Autodesk Inventor part; units mm, degrees
ref_plane "YZ Plane" through (0, 0, 0) normal (1, 0, 0) x (0, 1, 0)
ref_plane "XZ Plane" through (0, 0, 0) normal (0, 1, 0) x (-1, 0, 0)
ref_plane "XY Plane" through (0, 0, 0) normal (0, 0, 1) x (1, 0, 0)
sketch "Sketch1" plane through (0, 0, 0) normal (1, 0, 0) x (0, 1, 0)
  line L0 (0, 0) -> (3.175, 0)
  line L1 (3.175, 0) -> (3.175, -21.59)
  line L2 (3.175, -21.59) -> (0, -21.59)
  line L3 (0, -21.59) -> (0, 0)
  line L4 (0, 0) -> (29.591, 0)
  line L5 (29.591, 0) -> (29.591, -3.175)
  line L6 (29.591, -3.175) -> (0, -3.175)
  line L7 (0, -3.175) -> (0, 0)
  line L8 (29.591, 0) -> (26.416, 0)
  line L9 (26.416, 0) -> (26.416, -58.42)
  line L10 (26.416, -58.42) -> (29.591, -58.42)
  line L11 (29.591, -58.42) -> (29.591, 0)
  dimension "d0" = 3.175
  dimension "d1" = 21.59
  dimension "d4" = 3.175
  dimension "d5" = 29.591
  dimension "d6" = 3.175
  dimension "d7" = 58.42
extrude "Extrusion1" add sketch "Sketch1" along normal blind 12.7
sketch "Sketch2" plane through (0, 3.175, -3.175) normal (0, 0, -1) x (-1, 0, 0)
  circle A0 centre (-4.5212, 15.8052) radius 1.3589
  circle A1 centre (-4.5212, 6.1786) radius 1.3589
  line L0 (-12.7, 0) -> (-12.7, 23.241)
  point P0 (0, -3.175)
  dimension "d8" = 2.7178
  dimension "d9" = 2.7178
  dimension "d10" = 8.1788
  dimension "d11" = 8.1788
  dimension "d12" = 9.6266
extrude "Extrusion2" cut sketch "Sketch2" against normal blind 25.4
sketch "Sketch3" plane through (0, 3.175, -3.175) normal (0, 1, 0) x (1, 0, 0)
  circle A0 centre (6.35, 4.8202) radius 1.3589
  circle A1 centre (6.35, 14.8278) radius 1.3589
  line L0 (0, 18.415) -> (0, 0)
  point P0 (0, -3.175)
  dimension "d15" = 2.7178
  dimension "d16" = 2.7178
  dimension "d17" = 6.35
  dimension "d18" = 6.35
  dimension "d23" = 10.0076
extrude "Extrusion3" cut sketch "Sketch3" against normal blind 25.4
fillet "Fillet1" radius 3.175 1 edges at (6.35, 26.416, -3.175)
fillet "Fillet2" radius 2.286 1 edges at (6.35, 3.175, -3.175)
equation "\"d4\" = d0"
equation "\"d6\" = d0"
properties part number "U bracket"
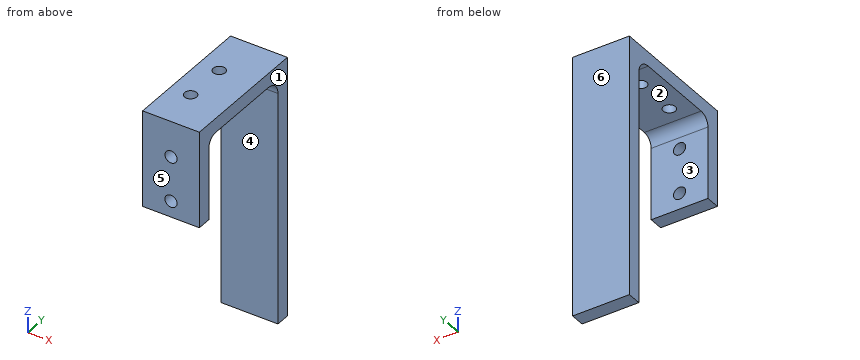
For this review, take the finished solid that the model builds, in its own axes (mm). Face numbers are marked on the shaded views. A direction names the side the tool comes from. Round coordinates to 2 decimals unless told otherwise and drop trailing zeros. Loops run counter-clockwise (first coordinate to the right, second up) from the corner with the lowest first, then second, coordinate; pieces in that order, holes last. Notation, with made-up numbers: (66.25, 36) - (122.25, 36) arc R27 ccw to (122.25, 61) - close; hole circle Ø5 at (-27, -2). An arc over 180 degrees is marked (long way). One line per question, with ' | ' between items.
Q1. Take a section at A-A (z = -10.5). Give the boundary of the cut face in (x, y) (3 decimals), and give its area (3 significant figures).
Taken from the geometry:
outline: (0, 0) - (12.7, 0) - (12.7, 3.175) - (0, 3.175) - close; (0, 26.416) - (12.7, 26.416) - (12.7, 29.591) - (0, 29.591) - close | area: 80.6 mm²
Q2. For pin 1 (6 mm diameter, centred on y = 6.5, z = -18.5, fed in from -X); pin 2 (2.5 mm diameter, centred on x = 5.5, y = 1.5, fed in from -Z); pin 3 (4 mm diameter, centred on x = 7, z = -44.5, fed in from -Y); pin 4 (4 mm diameter, centred on x = 7.5, y = 15, fed in from -Z) (3 decimals), all flat-tipped, find the tip position at first contact; note any pin that passes through.
Taken from the geometry:
pin 1: passes through | pin 2: stops at z = -21.59 | pin 3: stops at y = 26.42 | pin 4: stops at z = -3.175
Q3. Take a section at D-D (z = -38). Give the boundary of the cut face in (x, y).
Taken from the geometry:
outline: (0, 26.42) - (12.7, 26.42) - (12.7, 29.59) - (0, 29.59) - close
Q4. The part is to be moulded in two halves that separate along Y. For the marked faces 3, 4, 5 and 6, say which applies: released by +Y, released by -Y, zero draft, split by the parting line, or undercut.
Taken from the geometry:
face 3: undercut | face 4: undercut | face 5: released by -Y | face 6: released by +Y
Q5. Tool access review of the marked faces 1 and 2: name each direction out of +Z, -Z, +X, -X, +Y, -Y from which nothing blocks a thin tool from reaching the whole face with its end or side.
Taken from the geometry:
face 1: +Z, -Z, +X, +Y, -Y | face 2: -Z, +X, -X
Q6. Take a section at C-C (y = 6.25). Give the boundary of the cut face in (x, z) (3 decimals), and give its area (3 significant figures).
Taken from the geometry:
outline: (0, -3.175) - (12.7, -3.175) - (12.7, 0) - (0, 0) - close | area: 40.3 mm²
Q7. Take a section at B-B (x = 8.5). Give the boundary of the cut face in (y, z) (3 decimals), and give its area (3 significant figures).
Taken from the geometry:
outline: (0, -21.59) - (3.175, -21.59) - (3.175, -5.461) arc R2.286 cw to (5.461, -3.175) - (23.241, -3.175) arc R3.175 cw to (26.416, -6.35) - (26.416, -58.42) - (29.591, -58.42) - (29.591, 0) - (0, 0) - close | area: 331 mm²
Q8. For line 1 along Z through (x, y) = (6.35, 1.9); line 2 along Y through (x, z) = (10.25, -8) (3 decimals); line 3 along Z through (x, y) = (3.75, 1.75), list the stretches that pass through material, from the lowest coordinate up. Write a range as [from, to].
Taken from the geometry:
line 1: z = [-21.59, -19.36], [-16.64, -9.35], [-6.64, 0] | line 2: y = [0, 3.175], [26.416, 29.591] | line 3: z = [-21.59, 0]
